Job drawing, mm, ordinate dimensions from the low corner. One solid piece. A direction names the side the tool comes from. Round coordinates to 2 decimals unless told otherwise and drop trailing zeros. Order: outer loops, then holes, each group sorted by start corner. A loop starts at its lowest first (then second) coordinate and runs counter-clockwise, first axis right, second up. Notation, with made-up numbers: M -14.75,14.5 L -3.75,14.5 A33 cw -3.75,45.5 Z; hole C 4,8.25 d7. An arc over 180 degrees is marked long. Answer as a JSON object with one key per item and string values. Group by question number.
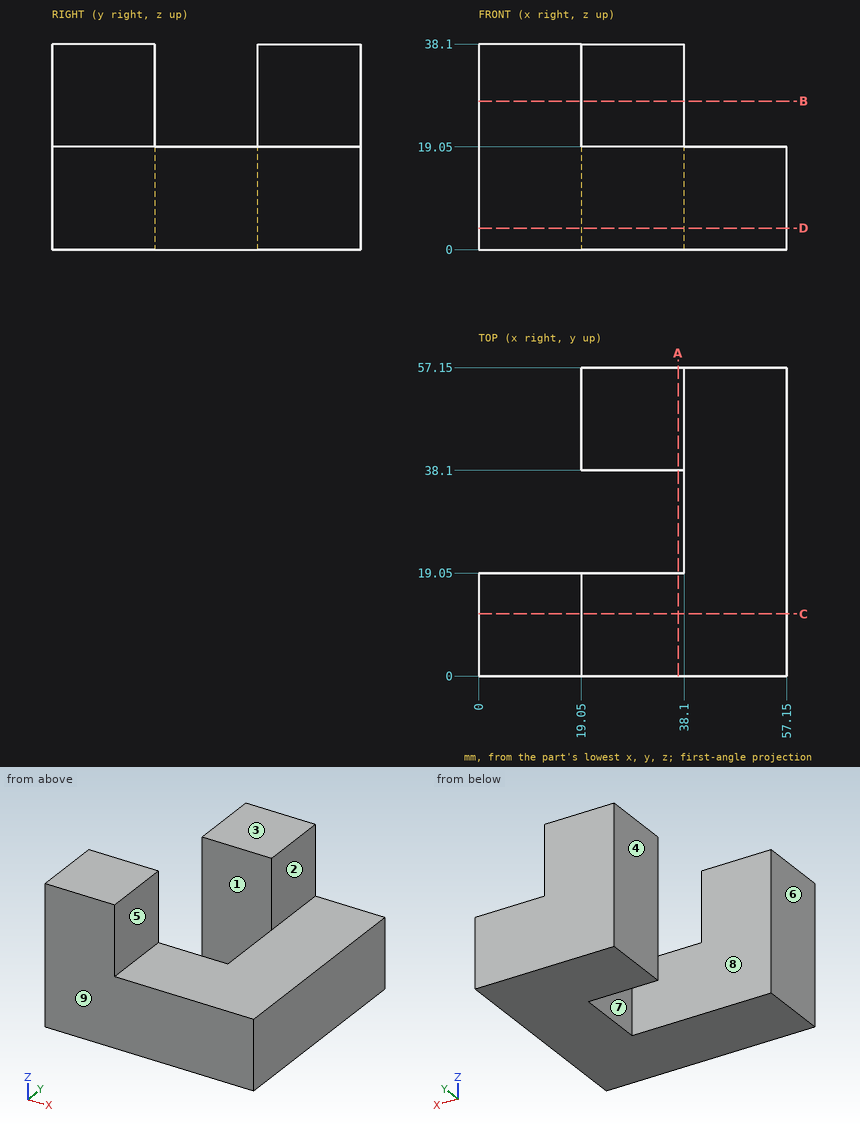
Item 1: Cut at A-A, the plane x = 37. Give the cut face in (y, z).
Item 2: Cut at C-C, the plane y = 11.5. Give the cut face in (x, z).
Item 3: Flat gauge pins, fed straight in: pin 1 Ø9.5 at (y, z) = (12, 24.5) entering from +X; pin 2 Ø1.5 at (x, z) = (10, 10.5) entering from +Y; pin 3 Ø4 at (y, z) = (38, 19.5) entering from -X. Where does each tip first touch, or does it go through?
Item 4: 3-axis set-ups, long thin cutter, end or side, ignore diameter. For the marked faces 1, 2, 3, 4 and 5: which of +Z, -Z, +X, -X, +Y, -Y reach the whole face in a straight line?
Item 5: Cut at B-B, the plane z = 27.5. Give the cut face in (x, y), and give its area (3 significant figures).
Item 6: Drill centre lines: line 1 (Y direction, x = 36, z = 30); line 2 (Y direction, x = 30, z = 14); line 3 (Y direction, x = 4, z = 11.5). Where is each one in solid material? Low to high. Write a range as [from, to].
Item 7: Cut at D-D, the plane z = 4. Give the cut face in (x, y).
Item 8: Two-plate mould, pull along Y, no slides. Class the marked faces 6, 7, 8 and 9: +Y half, -Y half, draft (parallel to the pull), parting line (faces both ways), or undercut.
Response values:
{
 "1": {"outline": "M 0,0 L 19.05,0 L 19.05,19.05 L 0,19.05 Z; M 38.1,0 L 57.15,0 L 57.15,38.1 L 38.1,38.1 Z"},
 "2": {"outline": "M 0,0 L 57.15,0 L 57.15,19.05 L 19.05,19.05 L 19.05,38.1 L 0,38.1 Z"},
 "3": {"pin 1": "x = 19.05", "pin 2": "y = 19.05", "pin 3": "x = 19.05"},
 "4": {"face 1": "+Z, -Z, -X", "face 2": "+Z, +X, +Y, -Y", "face 3": "+Z, +X, -X, +Y, -Y", "face 4": "+Z, -Z, -X, +Y", "face 5": "+Z, +X, -Y"},
 "5": {"outline": "M 0,0 L 19.05,0 L 19.05,19.05 L 0,19.05 Z; M 19.05,38.1 L 38.1,38.1 L 38.1,57.15 L 19.05,57.15 Z", "area": "726 mm^2"},
 "6": {"line 1": "[38.1, 57.15]", "line 2": "[0, 19.05], [38.1, 57.15]", "line 3": "[0, 19.05]"},
 "7": {"outline": "M 0,0 L 57.15,0 L 57.15,57.15 L 19.05,57.15 L 19.05,38.1 L 38.1,38.1 L 38.1,19.05 L 0,19.05 Z"},
 "8": {"face 6": "draft", "face 7": "undercut", "face 8": "undercut", "face 9": "-Y half"}
}
